Source: CAD feature listing. Evaluate the final solid. Frame: model axes, mm. A direction names the side the tool comes from. Round coordinates to 2 decimals unless told otherwise and drop trailing zeros. Write each loop counter-clockwise with the first axis right and the second up, starting at its lowest first coordinate (ties: lowest second). Pieces come first, ordered by that corner, then holes. Notation, with made-up numbers: M 45.5,81.5 L 83.5,81.5 A16 ccw 83.5,102.5 Z; hole C -15,24.5 d2. An arc over 180 degrees is marked long. Use a Markdown table: item, result.
```python
from build123d import *

# Parameters (mm, degrees)
SKETCH1_R           = 1.75
BASE_SHAPE_DEPTH    = 0.5
SKETCH2_W           = 3
SKETCH2_H           = 1
SKETCH2_W_2         = 1
SKETCH2_H_2         = 3
SKETCH2_W_3         = 2
SKETCH2_H_3         = 2
RX_SUPPORTS_DEPTH   = 1.75
SKETCH3_W           = 1.5
SKETCH3_H           = 5
CLIP_BASE_DEPTH     = 3.15
SKETCH4_W           = 1.85
SKETCH4_H           = 5
CLIP_TOP_DEPTH      = 1
CLIP_CHAMFER_REACH  = 41.42
SKETCH6_W           = 1.35
SKETCH6_H           = 1.35
BOSS_EXTRUDE1_DEPTH = 3.15


with BuildPart() as part:
    # Sketch1 → Base shape (new body)
    with BuildSketch(Plane.XY):
        with BuildLine():
            Line((18, -27.53772234), (18, 16))
            ThreePointArc((18, 16), (17.414213562, 17.414213562), (16, 18))
            Line((16, 18), (-16, 18))
            ThreePointArc((-16, 18), (-17.414213562, 17.414213562), (-18, 16))
            Line((-18, 16), (-18, -1.15))
            Line((-18, -1.15), (-16.2, -1.15))
            ThreePointArc((-16.2, -1.15), (-15.316116524, -1.516116524), (-14.95, -2.4))
            Line((-14.95, -2.4), (-14.95, -4.4))
            ThreePointArc((-14.95, -4.4), (-15.316116524, -5.283883476), (-16.2, -5.65))
            Line((-16.2, -5.65), (-18, -5.65))
            Line((-18, -5.65), (-18, -22.43))
            Line((-18, -22.43), (-11.95, -22.43))
            Line((-11.95, -22.43), (-11.95, -21.48))
            Line((-11.95, -21.48), (-10.95, -21.48))
            Line((-10.95, -21.48), (-10.95, -20.71))
            Line((-10.95, -20.71), (-4.01, -20.71))
            Line((-4.01, -20.71), (-4.01, -27.65))
            Line((-4.01, -27.65), (-10.95, -27.65))
            Line((-10.95, -27.65), (-10.95, -26.88))
            Line((-10.95, -26.88), (-11.95, -26.88))
            Line((-11.95, -26.88), (-11.95, -25.93))
            Line((-11.95, -25.93), (-18, -25.93))
            Line((-18, -25.93), (-18, -27.53772234))
            ThreePointArc((-18, -27.53772234), (-19.914525722, -31.468774411), (-16.5, -34.2))
            Line((-16.5, -34.2), (-2.3, -34.2))
            Line((-2.3, -34.2), (-2.3, -18))
            Line((-2.3, -18), (-1.2, -18))
            Line((-1.2, -18), (-1.2, -14.5))
            ThreePointArc((-1.2, -14.5), (-0.614213562, -13.085786438), (0.8, -12.5))
            Line((0.8, -12.5), (10.5, -12.5))
            ThreePointArc((10.5, -12.5), (11.914213562, -13.085786438), (12.5, -14.5))
            Line((12.5, -14.5), (12.5, -18))
            Line((12.5, -18), (13.6, -18))
            Line((13.6, -18), (13.6, -34.2))
            Line((13.6, -34.2), (16.5, -34.2))
            ThreePointArc((16.5, -34.2), (19.914525722, -31.468774411), (18, -27.53772234))
        make_face()
        with Locations((16.5, -30.7)):
            Circle(SKETCH1_R, mode=Mode.SUBTRACT)
        with Locations((15.25, 15.25)):
            Circle(SKETCH1_R, mode=Mode.SUBTRACT)
        with Locations((-15.25, -15.25)):
            Circle(SKETCH1_R, mode=Mode.SUBTRACT)
        with Locations((15.25, -15.25)):
            Circle(SKETCH1_R, mode=Mode.SUBTRACT)
        with Locations((-15.25, 15.25)):
            Circle(SKETCH1_R, mode=Mode.SUBTRACT)
        with BuildLine():
            ThreePointArc((-7.65, 14.9), (-8.4, 15.65), (-7.65, 16.4))
            Line((-7.65, 16.4), (-2.57, 16.4))
            ThreePointArc((-2.57, 16.4), (-1.82, 15.65), (-2.57, 14.9))
            Line((-2.57, 14.9), (-7.65, 14.9))
        make_face(mode=Mode.SUBTRACT)
        with Locations((-16.5, -30.7)):
            Circle(SKETCH1_R, mode=Mode.SUBTRACT)
    extrude(amount=BASE_SHAPE_DEPTH)

    # Sketch2 → RX supports (add)
    with BuildSketch(Plane.XY.offset(0.5)):
        with Locations((1.475, 6.95)):
            Rectangle(SKETCH2_W, SKETCH2_H)
        with Locations((-8.35, 1.45)):
            Rectangle(SKETCH2_W_2, SKETCH2_H_2)
        with Locations((-2.85, -5.2)):
            Rectangle(SKETCH2_W_3, SKETCH2_H_3)
        with Locations((11.3, 0.45)):
            Rectangle(SKETCH2_W_2, SKETCH2_H_2)
        with Locations((11.3, -5.25)):
            Rectangle(SKETCH2_W_2, SKETCH2_H_2)
    extrude(amount=RX_SUPPORTS_DEPTH)

    # Sketch3 → Clip base (add)
    with BuildSketch(Plane.XY.offset(0.5)):
        with Locations((-9.7, 1.95)):
            Rectangle(SKETCH3_W, SKETCH3_H)
        with Locations((12.65, 1.95)):
            Rectangle(SKETCH3_W, SKETCH3_H)
    extrude(amount=CLIP_BASE_DEPTH)

    # Sketch4 → Clip top (add)
    with BuildSketch(Plane.XY.offset(3.65)):
        with Locations((-9.525, 1.95)):
            Rectangle(SKETCH4_W, SKETCH4_H)
        with Locations((12.475, 1.95)):
            Rectangle(SKETCH4_W, SKETCH4_H)
    extrude(amount=CLIP_TOP_DEPTH)

    # Sketch5 → Clip chamfer (cut, up to next)
    with BuildSketch(Plane.XZ.offset(0.55), mode=Mode.PRIVATE) as clip_chamfer_sk1:
        Polygon((-8.6, 3.65), (-8.95, 4.65), (-8.6, 4.65), align=None)
    clip_chamfer_tool1 = extrude(clip_chamfer_sk1.sketch, amount=-CLIP_CHAMFER_REACH, mode=Mode.PRIVATE) & part.part
    # Sketch5 → Clip chamfer (cut, up to next)
    with BuildSketch(Plane.XZ.offset(0.55), mode=Mode.PRIVATE) as clip_chamfer_sk2:
        Polygon((11.55, 3.65), (11.9, 4.65), (11.55, 4.65), align=None)
    clip_chamfer_tool2 = extrude(clip_chamfer_sk2.sketch, amount=-CLIP_CHAMFER_REACH, mode=Mode.PRIVATE) & part.part
    add(clip_chamfer_tool1.solids().sort_by_distance((-8.716667, -0.55, 4.316667))[0], mode=Mode.SUBTRACT)
    add(clip_chamfer_tool2.solids().sort_by_distance((11.666667, -0.55, 4.316667))[0], mode=Mode.SUBTRACT)

    # Sketch6 → Boss-Extrude1 (add)
    with BuildSketch(Plane.XY.offset(0.5)):
        Polygon((-9.1, 17.2), (-7.75, 17.2), (-7.75, 18), (-10.45, 18), (-10.45, 16.4), (-9.1, 16.4), align=None)
        Polygon((13.4, 18), (10.7, 18), (10.7, 17.2), (12.05, 17.2), (12.05, 16.4), (13.4, 16.4), align=None)
        with Locations((12.725, -12.625)):
            Rectangle(SKETCH6_W, SKETCH6_H)
        Polygon((-9.1, -13.3), (-9.1, -11.95), (-10.45, -11.95), (-10.45, -14.65), (-7.75, -14.65), (-7.75, -13.3), align=None)
    extrude(amount=BOSS_EXTRUDE1_DEPTH)


solid = part.part
```
Q1. Section B-B on y = -30.7. Return loops of the section in (x, z).
Results are:
| item | result |
|---|---|
| outline | M -20,0 L -18.25,0 L -18.25,0.5 L -20,0.5 Z; M -14.75,0 L -2.3,0 L -2.3,0.5 L -14.75,0.5 Z; M 13.6,0 L 14.75,0 L 14.75,0.5 L 13.6,0.5 Z; M 18.25,0 L 20,0 L 20,0.5 L 18.25,0.5 Z |
Q2. Section C-C on z = 1.25. Give the number of separate pieces and of enclosed holes in the cut face, plus the area to 3 significant figures.
Results are:
| item | result |
|---|---|
| separate pieces | 11 |
| enclosed holes | 0 |
| area | 44.8 mm^2 |
Q3. Reachability of faces 1 (the cylindrical face through (11.9, -13.07, 0.25)), 2 (the flat face through (13, -0.55, 3)), 3 (the flat face through (13, 16.4, 2)), 4 (the flat face through (1, 6.45, 1)), 5 (the flat face through (11.72, 1.91, 4.14)) from +Z, -Z, +X, -X, +Y, -Y: full face, straight path, thin tool, end or side. Return the list, or none.
Results are:
| item | result |
|---|---|
| face 1 | +Z, -Z, -Y |
| face 2 | +Z, +X |
| face 3 | +Z, +X, -X |
| face 4 | +Z, +X, -X, -Y |
| face 5 | +Z, +Y, -Y |
Q4. Line query: L1, parallel to Y at x = -10, z = 3.1; L2, parallel to Y at x = 15.25, z = 0.2; L3, parallel to Y at x = -15.25, z = 0.45. Output: solid intervals per line, ascending.
Results are:
| item | result |
|---|---|
| L1 | -14.65 to -11.95, -0.55 to 4.45, 16.4 to 18 |
| L2 | -34.2 to -31.92, -29.48 to -17, -13.5 to 13.5, 17 to 18 |
| L3 | -34.2 to -31.92, -29.48 to -25.93, -22.43 to -17, -13.5 to -5.21, -1.59 to 13.5, 17 to 18 |
Q5. First-contact query: pin 1 Ø10 at (x, y) = (-1, -9) entering from +Z; pin 2 Ø1.1 at (y, z) = (-14, 1.5) entering from +X; pin 3 Ø8 at (x, y) = (-12.5, -0.5) entering from -Z; pin 4 Ø0.8 at (y, z) = (17, 2.5) entering from +X. Flat tips, straight axial feed; report the tip coordinate or a pass-through.
Results are:
| item | result |
|---|---|
| pin 1 | z = 2.25 |
| pin 2 | x = -7.75 |
| pin 3 | z = 0 |
| pin 4 | x = 13.4 |
Q6. Section D-D on y = 0.5. Return loops of the section in (x, z).
Results are:
| item | result |
|---|---|
| outline | M -18,0 L 18,0 L 18,0.5 L 13.4,0.5 L 13.4,4.65 L 11.9,4.65 L 11.55,3.65 L 11.9,3.65 L 11.9,0.5 L 11.8,0.5 L 11.8,2.25 L 10.8,2.25 L 10.8,0.5 L -7.85,0.5 L -7.85,2.25 L -8.85,2.25 L -8.85,0.5 L -8.95,0.5 L -8.95,3.65 L -8.6,3.65 L -8.95,4.65 L -10.45,4.65 L -10.45,0.5 L -18,0.5 Z |
Q7. Mould query, pull axis Y, two halves, no side actions, for faces 6 (the flat face through (11, 0, 2.25)), 7 (the flat face through (-3, -6.2, 1)), 8 (the cylindrical face through (16.272, -28.965, 0.246)). Classes: +Y half, -Y half, draft (parallel to the pull), parting line (faces both ways), or undercut.
Results are:
| item | result |
|---|---|
| face 6 | draft |
| face 7 | -Y half |
| face 8 | undercut |
Q8. Section A-A on y = -20. Return loops of the section in (x, z).
Results are:
| item | result |
|---|---|
| outline | M -18,0 L -2.3,0 L -2.3,0.5 L -18,0.5 Z; M 13.6,0 L 18,0 L 18,0.5 L 13.6,0.5 Z |
